Verification items for the finished model (mm, model axes). Face numbers are marked on the shaded views. A direction names the side the tool comes from. Give positions to 0.01 mm unless a question says otherwise; leave off trailing zeros. Write each loop counter-clockwise with the first axis right and the second up, starting at its lowest first coordinate (ties: lowest second). Pieces come first, ordered by that corner, then holes.
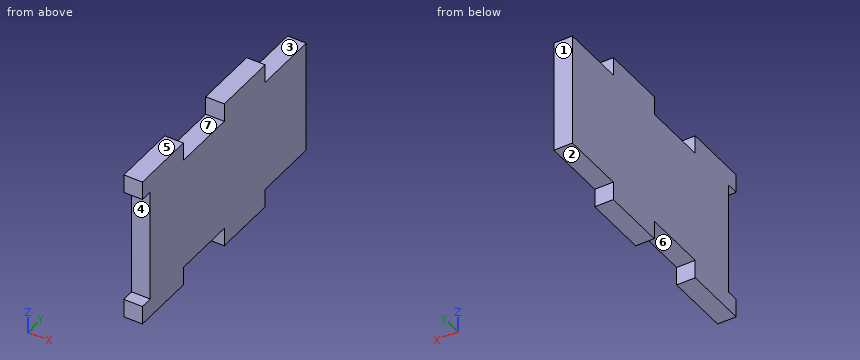
from build123d import *

# Parameters (mm, degrees)
BOSS_EXTRUDE1_DEPTH = 9.525
SKETCH2_W           = 58.42
SKETCH2_H           = 6.35
CUT_EXTRUDE1_DEPTH  = 46.99


with BuildPart() as part:
    # Sketch1 → Boss-Extrude1 (new body)
    with BuildSketch(Plane(origin=(0, 0, 0), x_dir=(0, 0, -1), z_dir=(1, 0, 0))):
        Polygon((9.525, -99.06), (0, -99.06), (0, -132.08), (77.47, -132.08), (77.47, -99.06), (67.945, -99.06), (67.945, -66.04), (77.47, -66.04), (77.47, -33.02), (67.945, -33.02), (67.945, 0), (9.525, 0), (9.525, -33.02), (0, -33.02), (0, -66.04), (9.525, -66.04), align=None)
    extrude(amount=BOSS_EXTRUDE1_DEPTH)

    # Sketch2 → Cut-Extrude1 (cut)
    with BuildSketch(Plane(origin=(9.525, 0, 0), x_dir=(0, 0, -1), z_dir=(1, 0, 0))):
        with Locations((38.735, -128.905)):
            Rectangle(SKETCH2_W, SKETCH2_H)
    extrude(amount=-CUT_EXTRUDE1_DEPTH, mode=Mode.SUBTRACT)


solid = part.part
Item 1: Sectioned sample at A-A on x = 5.75. Record the cut outline in (y, z) (3 decimals), then the cut area to 3 significant figures.
Answer key:
outline: (-132.08, -77.47) - (-99.06, -77.47) - (-99.06, -67.945) - (-66.04, -67.945) - (-66.04, -77.47) - (-33.02, -77.47) - (-33.02, -67.945) - (0, -67.945) - (0, -9.525) - (-33.02, -9.525) - (-33.02, 0) - (-66.04, 0) - (-66.04, -9.525) - (-99.06, -9.525) - (-99.06, 0) - (-132.08, 0) - (-132.08, -9.525) - (-125.73, -9.525) - (-125.73, -67.945) - (-132.08, -67.945) - close
area: 8,600 mm2
Item 2: Depth check by flat-ended pin: pin 1 (3 mm diameter, centred on x = 3, y = -89, fed in from -Z) (3 decimals); pin 2 (3 mm diameter, centred on x = 5.5, y = -86, fed in from +Z) (3 decimals); pin 3 (5 mm diameter, centred on x = 4, z = -72.5, fed in from +Y). Enter the tip coordinate at first touch or a pass-through.
Answer key:
pin 1: stops at z = -67.945
pin 2: stops at z = -9.525
pin 3: stops at y = -33.02
Item 3: Sectioned sample at C-C on y = -69. Record the cut outline in (x, z) (3 decimals), then the cut area to 3 significant figures.
Answer key:
outline: (0, -67.945) - (9.525, -67.945) - (9.525, -9.525) - (0, -9.525) - close
area: 556 mm2
Item 4: Release check for a two-part mould opening along Z. For the marked faces 1, 2, 3 and 4 record: released by +Z, released by -Z, zero draft, split by the parting line, or undercut.
Answer key:
face 1: zero draft
face 2: released by -Z
face 3: released by +Z
face 4: undercut
Item 5: Sectioned sample at B-B on z = -57. Record the cut outline in (x, y) (3 decimals), then the cut area to 3 significant figures.
Answer key:
outline: (0, -125.73) - (9.525, -125.73) - (9.525, 0) - (0, 0) - close
area: 1,200 mm2
Item 6: Scan lines: line 1 along Y through (x, z) = (1.5, -6); line 2 along Z through (x, y) = (3, -90) (3 decimals); line 3 along Y through (x, z) = (1.5, -47.5). Record each from-to range of solid material in increasing order.
Answer key:
line 1: y = -132.08 to -99.06, -66.04 to -33.02
line 2: z = -67.945 to -9.525
line 3: y = -125.73 to 0
Item 7: Set-up check for the marked faces 5, 6 and 7: record each of +Z, -Z, +X, -X, +Y, -Y from which the full face is reachable in a straight line by a thin tool's end or side.
Answer key:
face 5: +Z, +X, -X, +Y, -Y
face 6: -Z, +X, -X
face 7: +Z, +X, -X
